The listing builds one solid part. Answer for the finished solid, in the listing's coordinates (mm). A direction names the side the tool comes from. Round coordinates to 2 decimals unless told otherwise and drop trailing zeros. Order: outer loops, then holes, each group sorted by start corner. A loop starts at its lowest first (then second) coordinate and runs counter-clockwise, first axis right, second up. Notation, with made-up numbers: (39.25, 74) -> (46.25, 74) arc R24 cw to (46.25, 100) -> close; hole circle Ø11 at (-13.5, 73). An arc over 180 degrees is marked (long way). Return JSON: item names as keys, results as strings. Group by question number.
(1) Consider line 1 (Y direction, x = 16.25, z = 0); line 2 (Z direction, x = 9.75, y = -1.75); line 3 (Z direction, x = 15.5, y = 2.5). Determine where each line is inside the solid, lowest interval first. Write a range as [from, to].
(2) The part is cut by section C-C (x = 22.25). Determine the outline of the cut face in (y, z).
(3) The part is cut by section D-D (z = 10.75). Determine the outline of the cut face in (x, y), plus the area to 3 significant figures.
(4) The part is cut by section B-B (z = 5.5). Determine the outline of the cut face in (x, y).
(5) Which of the six approach directions +Z, -Z, +X, -X, +Y, -Y give full straight-line access (tool end or side, diameter ignored) to faces 1 (the face through (0, -12.3, 3.4)), 2 (the face through (23, -6, -6)), 3 (the face through (21, -3, -8))?
(6) The part is cut by section A-A (x = 11.5). Determine the outline of the cut face in (y, z), plus the area to 3 significant figures.
(7) Each of these flat-tipped pins is pushed along its axis until it touches: pin 1 (6 mm diameter, centred on x = 6, z = -11, fed in from +Y); pin 2 (2 mm diameter, centred on x = 23, z = 9, fed in from -Y); pin 3 (12 mm diameter, centred on x = 13, y = -8, fed in from -Z). Where does it stop, or does it pass through?
(8) Determine the mould class of faces 4 (the face through (23, 6, 6)), 5 (the face through (25, 0, 0)), 6 (the face through (12.68, -12.65, 8.06)) for opening direction Y: +Y half, -Y half, draft (parallel to the pull), parting line (faces both ways), or undercut.
from build123d import *
from build123d.topology import SkipClean

# Parameters (mm, degrees)
SKETCH1_W          = 25
SKETCH1_H          = 2.5
SKETCH2_W          = 17
SKETCH2_H          = 12.5
CUT_EXTRUDE1_DEPTH = 10
SKETCH4_R          = 12.5
SKETCH4_R_2        = 5
CUT_EXTRUDE2_DEPTH = 13
CUT_EXTRUDE3_DEPTH = 30.849623113


with BuildPart() as part:
    # Sketch1 → Revolve1 (revolve)
    with BuildSketch(Plane.XY, mode=Mode.PRIVATE) as revolve1_sk:
        with Locations((12.5, 13.75)):
            Rectangle(SKETCH1_W, SKETCH1_H)
    revolve(revolve1_sk.sketch.rotate(Axis((0, 0, 0), (1, 0, 0)), 90), axis=Axis((0, 0, 0), (1, 0, 0)))

    # Sketch2 → Revolve2 (revolve)
    with BuildSketch(Plane.XY, mode=Mode.PRIVATE) as revolve2_sk:
        with Locations((16.5, 6.25)):
            Rectangle(SKETCH2_W, SKETCH2_H)
    revolve(revolve2_sk.sketch.rotate(Axis((0, 0, 0), (1, 0, 0)), 90), axis=Axis((0, 0, 0), (1, 0, 0)))

    # Sketch3 → Cut-Extrude1 (cut)
    with BuildSketch(Plane.ZY.offset(-8)):
        with BuildLine():
            Line((0.829156198, 1.25), (0.829156198, -1.25))
            ThreePointArc((0.829156198, -1.25), (-1.5, 0), (0.829156198, 1.25))
        make_face()
    extrude(amount=-CUT_EXTRUDE1_DEPTH, mode=Mode.SUBTRACT)

    # Sketch4 → Cut-Extrude2 (cut)
    with BuildSketch(Plane.ZY.offset(-8)):
        Circle(SKETCH4_R)
        Circle(SKETCH4_R_2, mode=Mode.SUBTRACT)
    extrude(amount=-CUT_EXTRUDE2_DEPTH, mode=Mode.SUBTRACT)

    # Sketch5 → Cut-Extrude3 (cut, through all)
    with SkipClean():  # the faces are left unmerged after this step: merging them gives an invalid solid
        with BuildSketch(Plane.ZY.offset(-21)):
            with BuildLine():
                Line((12.5, 0), (5, 0))
                ThreePointArc((5, 0), (4.619397663, -1.913417162), (3.535533906, -3.535533906))
                Line((3.535533906, -3.535533906), (8.838834765, -8.838834765))
                ThreePointArc((8.838834765, -8.838834765), (11.548494156, -4.783542905), (12.5, 0))
            make_face()
            with BuildLine():
                Line((-12.5, 0), (-5, 0))
                ThreePointArc((-5, 0), (-4.619397663, 1.913417162), (-3.535533906, 3.535533906))
                Line((-3.535533906, 3.535533906), (-8.838834765, 8.838834765))
                ThreePointArc((-8.838834765, 8.838834765), (-11.548494156, 4.783542905), (-12.5, 0))
            make_face()
            with BuildLine():
                ThreePointArc((0, 5), (1.913417162, 4.619397663), (3.535533906, 3.535533906))
                Line((3.535533906, 3.535533906), (8.838834765, 8.838834765))
                ThreePointArc((8.838834765, 8.838834765), (4.783542905, 11.548494156), (0, 12.5))
                Line((0, 12.5), (0, 5))
            make_face()
            with BuildLine():
                Line((0, -12.5), (0, -5))
                ThreePointArc((0, -5), (-1.913417162, -4.619397663), (-3.535533906, -3.535533906))
                Line((-3.535533906, -3.535533906), (-8.838834765, -8.838834765))
                ThreePointArc((-8.838834765, -8.838834765), (-4.783542905, -11.548494156), (0, -12.5))
            make_face()
        extrude(amount=-CUT_EXTRUDE3_DEPTH, mode=Mode.SUBTRACT)


solid = part.part
Answer below:
{
 "1": {"line 1": "y = [-15, -12.5], [-5, -1.5], [1.5, 5], [12.5, 15]", "line 2": "z = [-14.9, -12.38], [-4.68, 4.68], [12.38, 14.9]", "line 3": "z = [-14.79, -12.25], [-4.33, 4.33], [12.25, 14.79]"},
 "2": {"outline": "circle Ø30 at (0, 0); hole (-12.5, 0) arc R12.5 ccw to (-8.84, -8.84) -> (-3.54, -3.54) arc R5 cw to (-5, 0) -> close; hole (-8.84, 8.84) -> (-3.54, 3.54) arc R5 cw to (0, 5) -> (0, 12.5) arc R12.5 ccw to start; hole (0, -12.5) arc R12.5 ccw to (8.84, -8.84) -> (3.54, -3.54) arc R5 cw to (0, -5) -> close; hole (3.54, 3.54) arc R5 cw to (5, 0) -> (12.5, 0) arc R12.5 ccw to (8.84, 8.84) -> close"},
 "3": {"outline": "(0, -10.46) -> (25, -10.46) -> (25, -6.38) -> (0, -6.38) -> close; (0, 6.38) -> (21, 6.38) -> (21, 0) -> (25, 0) -> (25, 10.46) -> (0, 10.46) -> close", "area": "230 mm²"},
 "4": {"outline": "(0, -13.96) -> (25, -13.96) -> (25, -5.5) -> (21, -5.5) -> (21, -11.22) -> (0, -11.22) -> close; (0, 11.22) -> (25, 11.22) -> (25, 13.96) -> (0, 13.96) -> close; (21, 0) -> (25, 0) -> (25, 5.5) -> (21, 5.5) -> close"},
 "5": {"face 1": "+Z, -Z, -X, +Y, -Y", "face 2": "+X, -X", "face 3": "-X"},
 "6": {"outline": "circle Ø30 at (0, 0); circle Ø10 at (0, 0); hole circle Ø25 at (0, 0); hole (-1.25, 0.83) arc R1.5 ccw (long way) to (1.25, 0.83) -> close", "area": "289 mm²"},
 "7": {"pin 1": "stops at y = 12.69", "pin 2": "stops at y = -12.69", "pin 3": "stops at z = -14.87"},
 "8": {"face 4": "undercut", "face 5": "draft", "face 6": "parting line"}
}
